```python
from build123d import *

# Parameters (mm, degrees)
BOSS_EXTRU_1_DEPTH      = 20
ENL_V_MAT_EXTRU_1_REACH = 63.847
ESQUISSE2_R             = 4.75
ENL_V_MAT_EXTRU_2_REACH = 64.881
ESQUISSE3_R             = 6
CONG_7_START            = -1
CONG_7_DEPTH            = 22
CONG_7_2_DEPTH          = 20
CONG_8_R                = 5
ENL_V_MAT_EXTRU_3_REACH = 64.881
ESQUISSE4_R             = 7.5
CONG_9_R                = 5
CONG_10_R               = 12


with BuildPart() as part:
    # Esquisse1 → Boss.-Extru.1 (new body)
    with BuildSketch(Plane(origin=(0, 0, 0), x_dir=(1, 0, 0), z_dir=(0, 1, 0))):
        Polygon((-30, 0), (-55, 0), (-55, 23), (55, 23), (55, 0), (25, 0), align=None)
        Polygon((28, 5), (28, 15), (10, 15), (10, 20), (-10, 20), (-10, 15), (-28, 15), (-28, 5), align=None, mode=Mode.SUBTRACT)
    extrude(amount=BOSS_EXTRU_1_DEPTH)

    # Esquisse2 → Enlèv. mat.-Extru.1 (cut, up to next)
    with BuildSketch(Plane.XY.offset(-20), mode=Mode.PRIVATE) as enl_v_mat_extru_1_sk1:
        with Locations((0, 10)):
            Circle(ESQUISSE2_R)
    enl_v_mat_extru_1_tool1 = extrude(enl_v_mat_extru_1_sk1.sketch, amount=-ENL_V_MAT_EXTRU_1_REACH, mode=Mode.PRIVATE) & part.part
    add(enl_v_mat_extru_1_tool1.solids().sort_by_distance((0, 10, -20))[0], mode=Mode.SUBTRACT)

    # Esquisse3 → Enlèv. mat.-Extru.2 (cut, up to next)
    with BuildSketch(Plane.XZ, mode=Mode.PRIVATE) as enl_v_mat_extru_2_sk1:
        with Locations(Location((45, -10, 0), (0, 0, 270))):
            Circle(ESQUISSE3_R)
    enl_v_mat_extru_2_tool1 = extrude(enl_v_mat_extru_2_sk1.sketch, amount=-ENL_V_MAT_EXTRU_2_REACH, mode=Mode.PRIVATE) & part.part
    # Esquisse3 → Enlèv. mat.-Extru.2 (cut, up to next)
    with BuildSketch(Plane.XZ, mode=Mode.PRIVATE) as enl_v_mat_extru_2_sk2:
        with Locations(Location((-45, -10, 0), (0, 0, 270))):
            Circle(ESQUISSE3_R)
    enl_v_mat_extru_2_tool2 = extrude(enl_v_mat_extru_2_sk2.sketch, amount=-ENL_V_MAT_EXTRU_2_REACH, mode=Mode.PRIVATE) & part.part
    add(enl_v_mat_extru_2_tool1.solids().sort_by_distance((45, 0, -10))[0], mode=Mode.SUBTRACT)
    add(enl_v_mat_extru_2_tool2.solids().sort_by_distance((-45, 0, -10))[0], mode=Mode.SUBTRACT)

    # Congé7: read off the stored shape, not the designer's step
    # Congé7 outline → Congé7 (cut)
    with BuildSketch(Plane(origin=(0, 0, 0), x_dir=(1, 0, 0), z_dir=(0, 1, 0)).offset(CONG_7_START)):
        with BuildLine():
            Line((-10, 15), (-10, 20))
            ThreePointArc((-10, 20), (-11.464466094, 16.464466094), (-15, 15))
            Line((-15, 15), (-10, 15))
        make_face()
        with BuildLine():
            Line((10, 15), (15, 15))
            ThreePointArc((15, 15), (11.464466094, 16.464466094), (10, 20))
            Line((10, 20), (10, 15))
        make_face()
    extrude(amount=CONG_7_DEPTH, mode=Mode.SUBTRACT)

    # Cong_7 2 outline → Cong_7 2 (add)
    with BuildSketch(Plane(origin=(0, 0, 0), x_dir=(1, 0, 0), z_dir=(0, 1, 0))):
        with BuildLine():
            ThreePointArc((-28, 10), (-26.535533906, 13.535533906), (-23, 15))
            Line((-23, 15), (-28, 15))
            Line((-28, 15), (-28, 10))
        make_face()
        with BuildLine():
            Line((28, 15), (23, 15))
            ThreePointArc((23, 15), (26.535533906, 13.535533906), (28, 10))
            Line((28, 10), (28, 15))
        make_face()
    extrude(amount=CONG_7_2_DEPTH)

    # Congé8
    cong_8_edges = [part.edges().sort_by_distance(p)[0] for p in [
        (-28, 10, -5),
        (28, 10, -5),
    ]]
    fillet(cong_8_edges, radius=CONG_8_R - 0.0001)  # a hair under: the kernel refuses the full size

    # Esquisse4 → Enlèv. mat.-Extru.3 (cut, up to next)
    with BuildSketch(Plane.XY, mode=Mode.PRIVATE) as enl_v_mat_extru_3_sk1:
        with Locations((0, 10)):
            Circle(ESQUISSE4_R)
    enl_v_mat_extru_3_tool1 = extrude(enl_v_mat_extru_3_sk1.sketch, amount=-ENL_V_MAT_EXTRU_3_REACH, mode=Mode.PRIVATE) & part.part
    add(enl_v_mat_extru_3_tool1.solids().sort_by_distance((0, 10, 0))[0], mode=Mode.SUBTRACT)

    # Congé9
    cong_9_edges = [part.edges().sort_by_distance(p)[0] for p in [
        (10, 10, -20),
        (-10, 10, -20),
    ]]
    fillet(cong_9_edges, radius=CONG_9_R)

    # Congé10
    # the kernel refuses this fillet: 12 mm, written as the material it takes off along each edge
    with BuildSketch(Plane(origin=(55, -30, -23), x_dir=(-1, 0, 0), z_dir=(0, 1, 0)), Plane(origin=(-55, -30, -23), x_dir=(0, 0, 1), z_dir=(0, 1, 0)), Plane(origin=(-55, -30, 0), x_dir=(1, 0, 0), z_dir=(0, 1, 0))) as cong_10_piece_1:
        with BuildLine():
            CenterArc((CONG_10_R, CONG_10_R), CONG_10_R, 180, 90)
            Line((0, CONG_10_R), (0, 0))
            Line((0, 0), (CONG_10_R, 0))
        make_face()
    extrude(amount=80, mode=Mode.SUBTRACT)
    with BuildSketch(Plane(origin=(55, -30, 0), x_dir=(-1, 0, 0), z_dir=(0, 1, 0))) as cong_10_piece_2:
        with BuildLine():
            CenterArc((CONG_10_R, -CONG_10_R), CONG_10_R, 90, 90)
            Line((0, -CONG_10_R), (0, 0))
            Line((0, 0), (CONG_10_R, 0))
        make_face()
    extrude(amount=80, mode=Mode.SUBTRACT)


solid = part.part
```
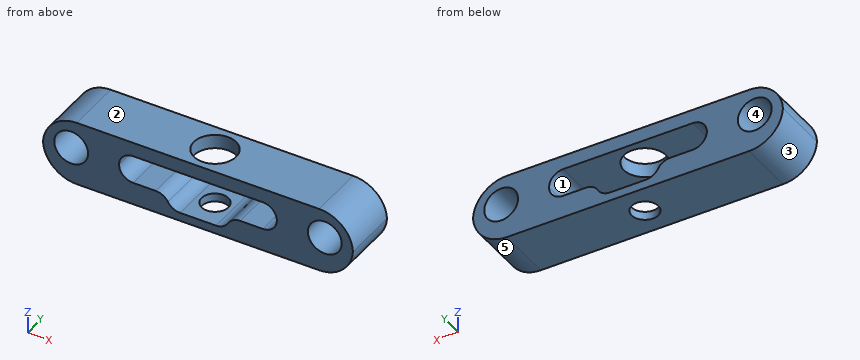
Geometry check sheet. Reference: the model listing, model coordinates, mm. Face numbers are marked on the shaded views. A direction names the side the tool comes from. Round coordinates to 2 decimals unless told otherwise and drop trailing zeros. Order: outer loops, then holes, each group sorted by start corner. A loop starts at its lowest first (then second) coordinate and runs counter-clockwise, first axis right, second up. Notation, with made-up numbers: M 25,31 L 51,31 A30 ccw 51,55 Z; hole C 83.25,10 d9. An arc over 180 degrees is marked long. Answer as CSV lines item,"result".
1) Sectioned sample at C-C on x = 0. Record the cut outline in (y, z).
Entries:
outline,"M 0,-23 L 5.25,-23 L 5.25,-20 L 0,-20 Z; M 0,-5 L 2.5,-5 L 2.5,0 L 0,0 Z; M 14.75,-23 L 20,-23 L 20,-20 L 14.75,-20 Z; M 17.5,-5 L 20,-5 L 20,0 L 17.5,0 Z"
2) Sectioned sample at B-B on x = 22. Record the cut outline in (y, z), and give its area (3 significant figures).
Entries:
outline,"M 0,-23 L 20,-23 L 20,-15 L 0,-15 Z; M 0,-5 L 20,-5 L 20,0 L 0,0 Z"
area,"260 mm2"
3) Sectioned sample at A-A on y = 10. Give the number of separate pieces and of enclosed holes in the cut face, and give its area (3 significant figures).
Entries:
separate pieces,"2"
enclosed holes,"2"
area,"1,430 mm2"
4) Tool access check on the marked faces 1 and 2. Record the directions out of +Z, -Z, +X, -X, +Y, -Y that give a thin tool (end or side, any length) a straight path to the whole face; none if there is none.
Entries:
face 1,"+Y, -Y"
face 2,"+Z, +X, -X, +Y, -Y"
5) Gauge pin test, flat ends, axial feed: pin 1 Ø12 at (x, y) = (0, 10) entering from +Z; pin 2 Ø6 at (y, z) = (2.5, -18) entering from -X; pin 3 Ø12 at (y, z) = (17.5, -19) entering from +X. Record the tip position at first contact, or that the pin passes through.
Entries:
pin 1,"z = -20"
pin 2,"x = -54.31"
pin 3,"x = 54.83"
6) Thickness scan on probe 1 along Z at (x, y) = (-15, 3); probe 2 along Z at (x, y) = (-0.5, 2); probe 3 along X at (y, z) = (7.75, -1.75). Record the ranges inside material, lowest first. Write a range as [from, to].
Entries:
probe 1,"[-23, -15], [-5, 0]"
probe 2,"[-23, -20], [-5, 0]"
probe 3,"[-49.24, -7.15], [7.15, 49.24]"
7) Mould release check, pull along X, two halves, no side actions. Record for the marked faces 3, 4 and 5: +X half, -X half, draft (parallel to the pull), parting line (faces both ways), or undercut.
Entries:
face 3,"-X half"
face 4,"undercut"
face 5,"+X half"
